```python
from build123d import *

# Parameters (mm, degrees)
EXTRUDE_1_DEPTH = 3


with BuildPart() as part:
    # 스케치1 → 보스-돌출1 (new body)
    with BuildSketch(Plane(origin=(0, 0, 0), x_dir=(0, 0, -1), z_dir=(1, 0, 0))):
        Polygon((51.8, 32), (51.8, 47), (51.8, 50), (46.8, 50), (46.8, 47), (41.8, 47), (27.155339059, 32.355339059), (25.034018716, 34.476659403), (7.356349186, 16.798989873), (9.47766953, 14.67766953), (-8.2, -3), (11.8, -3), (11.8, -8), (31.8, -8), (31.8, -3), (51.8, -3), (51.8, 12), (54.8, 12), (54.8, 32), align=None)
    extrude(amount=EXTRUDE_1_DEPTH)


solid = part.part
```
The listing builds one solid part. Answer for the finished solid, in the listing's coordinates (mm). A direction names the side the tool comes from. Give positions to 0.01 mm unless a question says otherwise; leave off trailing zeros. Write each loop counter-clockwise with the first axis right and the second up, starting at its lowest first coordinate (ties: lowest second). Pieces come first, ordered by that corner, then holes. Notation, with made-up numbers: (11.5, 13.25) - (32.5, 13.25) arc R30 cw to (32.5, 52.25) - close; hole circle Ø8 at (63.5, -3.5). An arc over 180 degrees is marked (long way). Use one line per item in the form item = value. Start each with the question number.
1) Flat-ended cylindrical pins translate along their axes: pin 1 Ø6 at (y, z) = (26.5, -43) entering from -X; pin 2 Ø1.5 at (x, z) = (1, -53) entering from -Y; pin 3 Ø1.5 at (x, y) = (1.5, 41.5) entering from +Z; pin 4 Ø1.5 at (x, z) = (2, -37) entering from -Y. Find the tip coordinate at first contact, or state that the pin passes through.
2) Find section B-B on z = -8.5. Determine the outline of the cut face in (x, y), plus the area to 3 significant figures.
3) Find section D-D on z = 2. Determine the outline of the cut face in (x, y), plus the area to 3 significant figures.
4) The mould has two halves that part along Y. Classify faces 4 (the face through (1, 12, -53)), 5 (the face through (1, 32, -53)), 6 (the face through (1, -6, -31.8)), 7 (the face through (1.479, 15.753, -8.402)): pulls with the +Y half, pulls with the -Y half, needs draft (parallel to the pull), parting line crosses it, or undercut.
5) Find section A-A on x = 0.9. Determine the outline of the cut face in (y, z).
6) A tool of negligible diameter and unlimited length cuts with its end or side. For faces 1 (the face through (1, 4, -51.8)), 2 (the face through (1, -5, -11.8)), 3 (the face through (1, 41, -51.8)), from which of +Z, -Z, +X, -X, +Y, -Y can it reach the whole face along a straight path? Write none if from no direction.
7) Find section C-C on y = 13. Determine the outline of the cut face in (x, z).
8) Consider line 1 along Z through (x, y) = (1.95, 33); line 2 along Y through (x, z) = (2.1, -8.5); line 3 along Z through (x, y) = (2.4, -5). Determine where each line is inside the solid, lowest interval first. Write a range as from..to.
Geometry results:
q1.pin_1 = 0
q1.pin_2 = 12
q1.pin_3 = -35.55
q1.pin_4 = -3
q2.outline = (0, -3) - (3, -3) - (3, 13.7) - (0, 13.7) - close; (0, 15.66) - (3, 15.66) - (3, 17.94) - (0, 17.94) - close
q2.area = 57.0 mm2
q3.outline = (0, -3) - (3, -3) - (3, 3.2) - (0, 3.2) - close
q3.area = 18.6 mm2
q4.face_4 = pulls with the -Y half
q4.face_5 = pulls with the +Y half
q4.face_6 = needs draft
q4.face_7 = undercut
q5.outline = (-8, -31.8) - (-3, -31.8) - (-3, -51.8) - (12, -51.8) - (12, -54.8) - (32, -54.8) - (32, -51.8) - (50, -51.8) - (50, -46.8) - (47, -46.8) - (47, -41.8) - (32.36, -27.16) - (34.48, -25.03) - (16.8, -7.36) - (14.68, -9.48) - (-3, 8.2) - (-3, -11.8) - (-8, -11.8) - close
q6.face_1 = -Z, +X, -X, -Y
q6.face_2 = +Z, +X, -X, -Y
q6.face_3 = -Z, +X, -X, +Y
q7.outline = (0, -54.8) - (3, -54.8) - (3, -7.8) - (0, -7.8) - close
q8.line_1 = -51.8..-27.8, -26.51..-23.56
q8.line_2 = -3..13.7, 15.66..17.94
q8.line_3 = -31.8..-11.8
